Model file for the job. Use its own axes, mm. Give positions to 0.01 mm unless a question says otherwise; leave off trailing zeros. Loops run counter-clockwise (first coordinate to the right, second up) from the corner with the lowest first, then second, coordinate; pieces in that order, holes last. Notation, with made-up numbers: M 48.5,65 L 73.5,65 A15 ccw 73.5,89 Z; hole C -39.75,74.25 d10. An arc over 180 degrees is marked long. Answer in a Markdown table with one row per item.
```python
from build123d import *

# Parameters (mm, degrees)
BOSS_EXTRUDE1_DEPTH = 100
FILLET1_R           = 30


with BuildPart() as part:
    # Sketch1 → Boss-Extrude1 (new body)
    with BuildSketch(Plane.XY):
        with BuildLine():
            Line((-331.6, 0), (-931.6, 0))
            ThreePointArc((-931.6, 0), (-806.789266166, 465.8), (-465.8, 806.789266166))
            Line((-465.8, 806.789266166), (-165.8, 287.174023895))
            ThreePointArc((-165.8, 287.174023895), (-287.174023895, 165.8), (-331.6, 0))
        make_face()
    extrude(amount=BOSS_EXTRUDE1_DEPTH)

    # Fillet1
    fillet1_edges = [part.edges().sort_by_distance(p)[0] for p in [
        (-806.789266166, 465.8, 100),
        (-631.6, 0, 100),
        (-287.174023895, 165.8, 100),
        (-631.6, 0, 0),
        (-806.789266166, 465.8, 0),
        (-315.8, 546.98164503, 0),
        (-287.174023895, 165.8, 0),
        (-331.6, 0, 50),
        (-931.6, 0, 50),
        (-465.8, 806.789266166, 50),
        (-165.8, 287.174023895, 50),
        (-315.8, 546.98164503, 100),
    ]]
    fillet(fillet1_edges, radius=FILLET1_R)


solid = part.part
```
Q1. Drop flat-ended pins along their axis: pin 1 (5 mm diameter, centred on x = -275.5, z = 21, fed in from +Y); pin 2 (1.5 mm diameter, centred on y = 509, z = 61, fed in from -X); pin 3 (12 mm diameter, centred on y = 577, z = 59.5, fed in from -X). Give the stop position or say it passes through.
Reported:
| item | result |
|---|---|
| pin 1 | y = 479 |
| pin 2 | x = -780.74 |
| pin 3 | x = -736.1 |
Q2. Saw through at A-A (z = 15). Give the cut face in (x, y), and give its area (3 significant figures).
Reported:
| item | result |
|---|---|
| outline | M -927.07,30.86 A25.98 ccw -901.1,4.02 L -360.35,4.02 A25.98 ccw -334.46,27.84 A335.62 cw -191.35,275.73 A25.98 ccw -183.66,310.07 L -454.03,778.37 A25.98 ccw -490.26,787.43 A927.58 ccw Z |
| area | 386,000 mm² |
Q3. Probe probe 1 along Y at (x, z) = (-266.5, 66); probe 2 along X at (y, z) = (413, 43); probe 3 along Y at (x, z) = (-423.5, 44). List the from-to ranges inside material, lowest first.
Reported:
| item | result |
|---|---|
| probe 1 | 197.32 to 461.59 |
| probe 2 | -835.05 to -238.45 |
| probe 3 | 0 to 733.52 |
